```python
from build123d import *

# Parameters (mm, degrees)
F0_W     = 215.9
F0_H     = 215.9
F1_DEPTH = 50.8
F2_W     = 60.96
F2_H     = 186.68595
F2_W_2   = 59.69
F2_W_3   = 57.038961
F2_H_2   = 60.011442
F3_DEPTH = 19.05
F4_W     = 88.9
F4_H     = 38.1
F5_DEPTH = 12.7
F7_DEPTH = 78.74


with BuildPart() as f1:
    # F0 (on Top) → F1 (new body)
    with BuildSketch(Plane.XY):
        Rectangle(F0_W, F0_H)
    extrude(amount=F1_DEPTH)

    # F2 (on face) → F3 (cut)
    with BuildSketch(Plane.XY.offset(50.8)):
        with Locations((-61.690293, 0)):
            Rectangle(F2_W, F2_H)
        with Locations((1.960519, 0)):
            Rectangle(F2_W_2, F2_H)
        with Locations((63.650813, 63.337254)):
            Rectangle(F2_W_3, F2_H_2)
        with Locations((63.650813, 0)):
            Rectangle(F2_W_3, F2_H_2)
        with Locations((63.650813, -63.337254)):
            Rectangle(F2_W_3, F2_H_2)
    extrude(amount=-F3_DEPTH, mode=Mode.SUBTRACT)

    # F4 (on face) → F5 (cut)
    with BuildSketch(Plane(origin=(0, 0, 0), x_dir=(1, 0, 0), z_dir=(0, 0, -1))):
        Rectangle(F4_W, F4_H)
    extrude(amount=-F5_DEPTH, mode=Mode.SUBTRACT)

    # F6 (on face) → F7 (cut)
    with BuildSketch(Plane.XZ.offset(-19.05)):
        Polygon((-32.131, 0), (0, 0), (32.131, 0), (39.4208, 12.7), (-39.4208, 12.7), align=None)
    extrude(amount=-F7_DEPTH, mode=Mode.SUBTRACT)


solid = f1.part
```
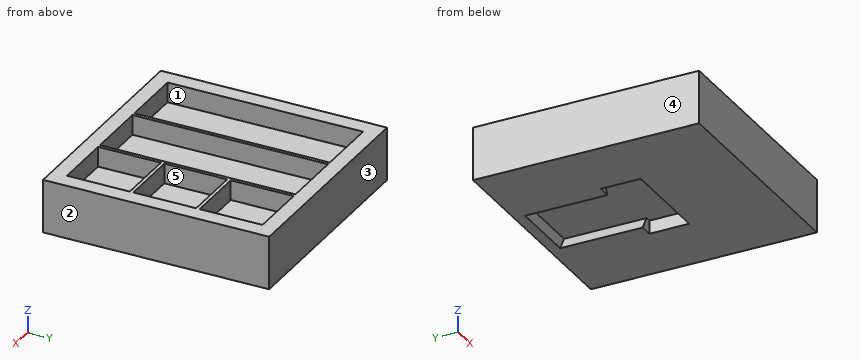
Geometry check sheet. Reference: the model listing, model coordinates, mm. Face numbers are marked on the shaded views. A direction names the side the tool comes from. Coordinates: 2 decimals unless noted, no trailing zeros. Order: outer loops, then holes, each group sorted by start corner. A loop starts at its lowest first (then second) coordinate and runs counter-clockwise, first axis right, second up.
Item 1: Mould release check, pull along Y, two halves, no side actions. Record for the marked faces 1, 2 and 3: released by +Y, released by -Y, zero draft, split by the parting line, or undercut.
Item 2: Section check B-B (y = -37.5). Enter the section's corners in (x, z).
Item 3: Section check D-D (x = -73.5). Enter the section's corners in (y, z), plus the area to 3 significant figures.
Item 4: Section check A-A (z = 43.5). Enter the section's corners in (x, y).
Item 5: Section check C-C (x = 48). Enter the section's corners in (y, z), plus the area to 3 significant figures.
Item 6: Depth check by flat-ended pin: pin 1 (18 mm diameter, centred on x = 15.5, y = -35, fed in from +Z). Enter the tip coordinate at first touch or a pass-through.
Item 7: Tool access check on the marked faces 4 and 5. Record the directions out of +Z, -Z, +X, -X, +Y, -Y that give a thin tool (end or side, any length) a straight path to the whole face; none if there is none.
Item 8: Scan lines: line 1 along X through (y, z) = (-19, 33.5); line 2 along Y through (x, z) = (-80, 44); line 3 along X through (y, z) = (-1.5, 8). Record each from-to range of solid material in increasing order.
Check sheet entries:
1. face 1: undercut
1. face 2: zero draft
1. face 3: released by +Y
2. outline: (-107.95, 0) - (107.95, 0) - (107.95, 50.8) - (92.17, 50.8) - (92.17, 31.75) - (35.13, 31.75) - (35.13, 50.8) - (31.81, 50.8) - (31.81, 31.75) - (-27.88, 31.75) - (-27.88, 50.8) - (-31.21, 50.8) - (-31.21, 31.75) - (-92.17, 31.75) - (-92.17, 50.8) - (-107.95, 50.8) - close
3. outline: (-107.95, 0) - (107.95, 0) - (107.95, 50.8) - (93.34, 50.8) - (93.34, 31.75) - (-93.34, 31.75) - (-93.34, 50.8) - (-107.95, 50.8) - close
3. area: 7,410 mm2
4. outline: (-107.95, -107.95) - (107.95, -107.95) - (107.95, 107.95) - (-107.95, 107.95) - close; hole (-92.17, -93.34) - (-31.21, -93.34) - (-31.21, 93.34) - (-92.17, 93.34) - close; hole (-27.88, -93.34) - (31.81, -93.34) - (31.81, 93.34) - (-27.88, 93.34) - close; hole (35.13, -93.34) - (92.17, -93.34) - (92.17, -33.33) - (35.13, -33.33) - close; hole (35.13, -30.01) - (92.17, -30.01) - (92.17, 30.01) - (35.13, 30.01) - close; hole (35.13, 33.33) - (92.17, 33.33) - (92.17, 93.34) - (35.13, 93.34) - close
5. outline: (-107.95, 0) - (107.95, 0) - (107.95, 50.8) - (93.34, 50.8) - (93.34, 31.75) - (33.33, 31.75) - (33.33, 50.8) - (30.01, 50.8) - (30.01, 31.75) - (-30.01, 31.75) - (-30.01, 50.8) - (-33.33, 50.8) - (-33.33, 31.75) - (-93.34, 31.75) - (-93.34, 50.8) - (-107.95, 50.8) - close
5. area: 7,540 mm2
6. pin 1: stops at z = 31.75
7. face 4: +Z, -Z, -X, +Y, -Y
7. face 5: +Z
8. line 1: x = -107.95 to -92.17, -31.21 to -27.88, 31.81 to 35.13, 92.17 to 107.95
8. line 2: y = -107.95 to -93.34, 93.34 to 107.95
8. line 3: x = -107.95 to -44.45, 44.45 to 107.95
